The model under review builds one solid part; all positions refer to its coordinate system, in mm. A direction names the side the tool comes from. Coordinates: 2 decimals unless noted, no trailing zeros. Write each loop counter-clockwise with the first axis right and the second up, starting at its lowest first coordinate (ties: lowest second). Pieces come first, ordered by that corner, then holes. Notation, with made-up numbers: (53.25, 71) - (64.25, 71) arc R9 ccw to (64.25, 80) - close; hole circle Ø6 at (48, 67). An arc over 180 degrees is marked (long way). Put each result on its own line as item: value. Start each with the question number.
Item 1: Machinability: for faces 4 (the face through (-31.399, -13, 24)), 5 (the face through (0, -13, 51)), 6 (the face through (22.561, -13, -27)), which of the approach directions +Z, -Z, +X, -X, +Y, -Y give a long, thin tool a straight path to every point of the face, cutting with its end or side? Answer none if there is none.
Item 2: Mouldability with a two-part tool opening along X and no side actions: class faces 1 (the face through (-24, -13, 51.867)), 2 (the face through (-17.677, -13, 14)), 3 (the face through (41.866, -13, 13)) as pulls with the +X half, pulls with the -X half, needs draft (parallel to the pull), parting line crosses it, or undercut.
Item 3: Consider section D-D on y = -10. State how many separate pieces and enclosed holes the cut face has, then the cut area to 3 significant figures.
Item 4: For pin 1 (6 mm diameter, centred on x = 33.5, y = -9.5, fed in from -Z); pin 2 (5 mm diameter, centred on x = 16, y = -11, fed in from +Z); pin 3 (4 mm diameter, centred on y = -19, z = 47, fed in from +X), all flat-tipped, find the tip position at first contact; note any pin that passes through.
Item 5: Consider section C-C on x = -2. Give the boundary of the cut face in (y, z).
Item 6: Consider section A-A on z = 5. Give the boundary of the cut face in (x, y).
Item 7: To check wall thickness, follow L1, parallel to X at y = -13, z = 21.5; L2, parallel to Z at x = -2, y = -8.25; L3, parallel to Z at x = 15, y = -23.25. State the ranges of each line that lie inside material, in increasing order. Write a range as [from, to].
Item 8: Consider section B-B on z = 23. Give the boundary of the cut face in (x, y), then the cut area to 3 significant figures.
```python
from build123d import *

# Parameters (mm, degrees)
F0_W     = 3.7213962059
F0_H     = 17.6766254008
F0_H_2   = 3.7213973701
F0_W_2   = 3.2562217675
F0_H_3   = 20.467672497
F0_W_3   = 3.9539821446
F0_H_4   = 23.2587195933
F0_W_4   = 16.9788654894
F0_W_5   = 5.3495056927
F0_H_5   = 2.0932843909
F0_W_6   = 0.4651769996
F0_H_6   = 8.6057269946
F0_W_7   = 14.1878202558
F0_H_7   = 29.5385746285
F1_DEPTH = 25.4


with BuildPart() as f1:
    # F0 (on Front) → F1 (new body)
    with BuildSketch(Plane.XZ):
        Polygon((0, -12.7922967076), (0, 0), (-5.8146808296, 0), (-9.3034878373, 0), (-13.7226451188, 0), (-13.7226451188, -23.2587195933), (-17.6766272634, -23.2587195933), (-17.6766272634, -33.2599692047), (6.7450278439, -33.2599692047), (6.7450278439, -12.7922967076), align=None)
        Polygon((-13.7226451188, 28.1430520117), (0, 28.1430520117), (0, 45.8196774125), (0, 49.5410747826), (-35.1206697524, 49.5410747826), (-35.1206697524, 38.1443016231), (-31.3992723823, 38.1443016231), (-31.3992723823, 35.3532582521), (-13.7226451188, 35.3532582521), align=None)
        with Locations((1.860698103, 36.9813647121)):
            Rectangle(F0_W, F0_H)
        with Locations((1.860698103, 47.6803760976)):
            Rectangle(F0_W, F0_H_2)
        Polygon((-17.6766272634, 28.1430520117), (-13.7226451188, 28.1430520117), (-13.7226451188, 35.3532582521), (-31.3992723823, 35.3532582521), (-31.3992723823, 8.6057269946), (-34.6554927528, 8.6057269946), (-34.6554927528, 0), (-17.6766272634, 0), align=None)
        Polygon((3.7213962059, 45.8196774125), (3.7213962059, 28.1430520117), (10.0012496114, 28.1430520117), (10.0012496114, 2.558459295), (17.2114521265, 2.558459295), (17.2114521265, 40.9353487194), (29.0734022856, 40.9353487194), (29.0734022856, 45.8196774125), align=None)
        with Locations((8.3731387276, -23.0261329561)):
            Rectangle(F0_W_2, F0_H_3)
        with Locations((-15.6996361911, -11.6293597966)):
            Rectangle(F0_W_3, F0_H_4)
        Polygon((-35.1206697524, 49.5410747826), (0, 49.5410747826), (0, 51.8669486046), (-49.3084900081, 51.8669486046), (-49.3084900081, 38.1443016231), (-35.1206697524, 38.1443016231), align=None)
        Polygon((17.2114521265, -12.7922967076), (10.0012496114, -12.7922967076), (10.0012496114, -33.2599692047), (6.7450278439, -33.2599692047), (6.7450278439, -38.1443016231), (22.5609578192, -38.1443016231), (22.5609578192, -14.8855810985), (17.2114521265, -14.8855810985), align=None)
        with Locations((-26.1660600081, -11.6293597966)):
            Rectangle(F0_W_4, F0_H_4)
        with Locations((19.8862049729, -13.8389389031)):
            Rectangle(F0_W_5, F0_H_5)
        with Locations((-34.8880812526, 4.3028634973)):
            Rectangle(F0_W_6, F0_H_6)
        with Locations((-42.2145798802, 23.3750143088)):
            Rectangle(F0_W_7, F0_H_7)
        Polygon((41.8656989932, 40.9353487194), (29.0734022856, 40.9353487194), (29.0734022856, -12.7922967076), (22.5609578192, -12.7922967076), (22.5609578192, -14.8855810985), (41.8656989932, -14.8855810985), align=None)
        Polygon((29.0734022856, -12.7922967076), (29.0734022856, 40.9353487194), (17.2114521265, 40.9353487194), (17.2114521265, 2.558459295), (22.5609578192, 2.558459295), (22.5609578192, -12.7922967076), align=None)
        with Locations((-42.2145798802, 4.3028634973)):
            Rectangle(F0_W_7, F0_H_6)
    extrude(amount=F1_DEPTH)


solid = f1.part
```
Report:
1. face 4: +Y, -Y
1. face 5: +Z, +X, +Y, -Y
1. face 6: -Z, +X, +Y, -Y
2. face 1: needs draft
2. face 2: undercut
2. face 3: pulls with the +X half
3. separate pieces: 1
3. enclosed holes: 2
3. area: 5,320 mm²
4. pin 1: z = -14.89
4. pin 2: z = 45.82
4. pin 3: x = 29.07
5. outline: (-25.4, -33.26) - (0, -33.26) - (0, 0) - (-25.4, 0) - close; (-25.4, 28.14) - (0, 28.14) - (0, 51.87) - (-25.4, 51.87) - close
6. outline: (-49.31, -25.4) - (-17.68, -25.4) - (-17.68, 0) - (-49.31, 0) - close; (10, -25.4) - (41.87, -25.4) - (41.87, 0) - (10, 0) - close
7. L1: [-49.31, -35.12], [-31.4, -17.68], [10, 41.87]
7. L2: [-33.26, 0], [28.14, 51.87]
7. L3: [-38.14, -12.79], [2.56, 45.82]
8. outline: (-49.31, -25.4) - (-35.12, -25.4) - (-35.12, 0) - (-49.31, 0) - close; (-31.4, -25.4) - (-17.68, -25.4) - (-17.68, 0) - (-31.4, 0) - close; (10, -25.4) - (41.87, -25.4) - (41.87, 0) - (10, 0) - close
8. area: 1,520 mm²
